Read the model definition and answer for the solid it produces. Units are mm, in the model's axes. Round coordinates to 2 decimals unless told otherwise and drop trailing zeros. Loops run counter-clockwise (first coordinate to the right, second up) from the corner with the lowest first, then second, coordinate; pieces in that order, holes last. Notation, with made-up numbers: (6.25, 10.5) - (34.25, 10.5) arc R13 cw to (34.25, 30.5) - close; hole circle Ø9 at (2.5, 7). An arc over 180 degrees is marked (long way). Use one line per item in the form item = value. Start each with the question number.
Autodesk Inventor part; units mm, degrees
ref_plane "YZ Plane" through (0, 0, 0) normal (1, 0, 0) x (0, 1, 0)
ref_plane "XZ Plane" through (0, 0, 0) normal (0, 1, 0) x (-1, 0, 0)
ref_plane "XY Plane" through (0, 0, 0) normal (0, 0, 1) x (1, 0, 0)
sketch "Skizze1" plane through (0, 0, 0) normal (0, 0, 1) x (1, 0, 0)
  line L0 (0, 0) -> (20, 0)
  line L1 (20, 0) -> (20, 20)
  line L2 (20, 20) -> (0, 20)
  line L3 (0, 20) -> (0, 0)
  dimension "d0" = 20
  dimension "d1" = 20
extrude "Extrusion1" add sketch "Skizze1" along normal blind 2
sketch "Skizze2" plane through (0, 0, 2) normal (0, 0, 1) x (1, 0, 0)
  line L0 (0, 0) -> (0, 20)
  line L1 (20, 20) -> (20, 0)
  line L2 (0, 20) -> (20, 20)
  line L3 (0, 15) -> (20, 15)
  point P0 (5, 15)
  point P1 (15, 15)
  dimension "d4" = 5
  dimension "d5" = 5
  dimension "d6" = 10
hole "Bohrung1" at (5, 15, 2) at (15, 15, 2) direction (0, 0, -1) diameter 3.4 end through all
sketch "Skizze3" plane through (0, 0, 2) normal (0, 0, 1) x (1, 0, 0)
  line L0 (0, 0) -> (0, 20)
  line L1 (20, 0) -> (0, 0)
  line L2 (20, 20) -> (20, 0)
  line L3 (0, 5) -> (20, 5)
  line L4 (10, 0) -> (10, 7.2656)
  point P0 (6, 5)
  point P1 (14, 5)
  dimension "d14" = 8
  dimension "d15" = 5
hole "Bohrung2" at (6, 5, 2) at (14, 5, 2) direction (0, 0, -1) diameter 2.459 end through all
properties part number "13_0204_071"
1) A cutting plane is placed at C-C on x = 15. Write down the section's boundary in (y, z).
2) Straight lines are drawn through the part: line 1 (X direction, y = 5, z = 1.65); line 2 (Y direction, x = 5, z = 1.5); line 3 (X direction, y = 15, z = 0.5). For each, find the intervals that lie inside material, in ascending order. Write a range as from..to.
3) A cutting plane is placed at B-B on z = 1.15. Write down the section's boundary in (x, y).
4) Determine the mould class of faces 1 (the cylindrical face through (6.748, 5.976, 0.986)), 2 (the flat face through (10, 0, 1)), 3 (the flat face through (0, 10, 1)) for opening direction Y: +Y half, -Y half, draft (parallel to the pull), parting line (faces both ways), or undercut.
5) A cutting plane is placed at A-A on y = 5. Write down the section's boundary in (x, z), plus the area to 3 significant figures.
Checks:
q1.outline = (0, 0) - (4.28, 0) - (4.28, 2) - (0, 2) - close; (5.72, 0) - (13.3, 0) - (13.3, 2) - (5.72, 2) - close; (16.7, 0) - (20, 0) - (20, 2) - (16.7, 2) - close
q2.line_1 = 0..4.77, 7.23..12.77, 15.23..20
q2.line_2 = 0..4.28, 5.72..13.3, 16.7..20
q2.line_3 = 0..3.3, 6.7..13.3, 16.7..20
q3.outline = (0, 0) - (20, 0) - (20, 20) - (0, 20) - close; hole circle Ø3.4 at (5, 15); hole circle Ø2.46 at (6, 5); hole circle Ø2.46 at (14, 5); hole circle Ø3.4 at (15, 15)
q4.face_1 = undercut
q4.face_2 = -Y half
q4.face_3 = draft
q5.outline = (0, 0) - (4.77, 0) - (4.77, 2) - (0, 2) - close; (7.23, 0) - (12.77, 0) - (12.77, 2) - (7.23, 2) - close; (15.23, 0) - (20, 0) - (20, 2) - (15.23, 2) - close
q5.area = 30.2 mm²
